Can you work these out from the model? Positions are in its coordinate system, mm. Coordinates: 2 decimals unless noted, no trailing zeros. Write each loop counter-clockwise with the first axis right and the second up, starting at its lowest first coordinate (ties: lowest second). Pieces come first, ordered by that corner, then holes. Notation, with made-up numbers: (83, 49.25) - (105, 49.25) arc R24 cw to (105, 70.25) - close; hole circle Ø5 at (31, 73). An arc over 180 degrees is marked (long way). Use one line per item in the form item = value. Start each with the question number.
(1) If we section it at C-C on y = -127.5: Please give me the cut outline in (x, z), then the cut area to 3 significant figures.
(2) If we section it at B-B on z = 0: Please give me the cut outline in (x, y), then the cut area to 3 significant figures.
(3) If we section it at A-A on x = 0: Please give me the cut outline in (y, z), then the cut area to 3 significant figures.
(4) If I drill on probe 1 along Z at (x, y) = (15, -39.45); probe 2 along Y at (x, z) = (-16.5, 14.5); probe 3 along Z at (x, y) = (-1.5, -140), over which ranges is the centre line in solid material (lowest first)? Write a range as from..to.
(5) For pin 1 Ø4 at (x, y) = (4, -64) entering from -Z; pin 2 Ø5 at (x, z) = (-16, -15) entering from +Y; pin 3 Ø2.5 at (x, z) = (-16, -15.5) entering from -Y; pin 4 Ø0.9 at (x, z) = (15.5, -15) entering from -Y, each with a flat end and sliding along its axis, tell me the tip position at first contact or that it passes through.
```python
from build123d import *

# Parameters (mm, degrees)
F0_W     = 42
F0_H     = 42
F1_DEPTH = 40
F2_R     = 4
F3_DEPTH = 325
F4_R     = 1.5
F5_DEPTH = 2


with BuildPart() as f1:
    # F0 (on Front) → F1 (new body)
    with BuildSketch(Plane.XZ):
        Rectangle(F0_W, F0_H)
    extrude(amount=F1_DEPTH)

    # F2 (on face) → F3 (join)
    with BuildSketch(Plane.XZ.offset(40)):
        Circle(F2_R)
    extrude(amount=F3_DEPTH)

    # F4 (on face) → F5 (cut)
    with BuildSketch(Plane.XZ.offset(40)):
        with Locations((-16, -15)):
            Circle(F4_R)
        with BuildLine():
            ThreePointArc((-17.5, 16), (-16, 14.5), (-14.5, 16))
            ThreePointArc((-14.5, 16), (-16, 17.5), (-17.5, 16))
        make_face()
        with Locations((15, -15)):
            Circle(F4_R)
        with Locations((15, 16)):
            Circle(F4_R)
    extrude(amount=-F5_DEPTH, mode=Mode.SUBTRACT)


solid = f1.part
```
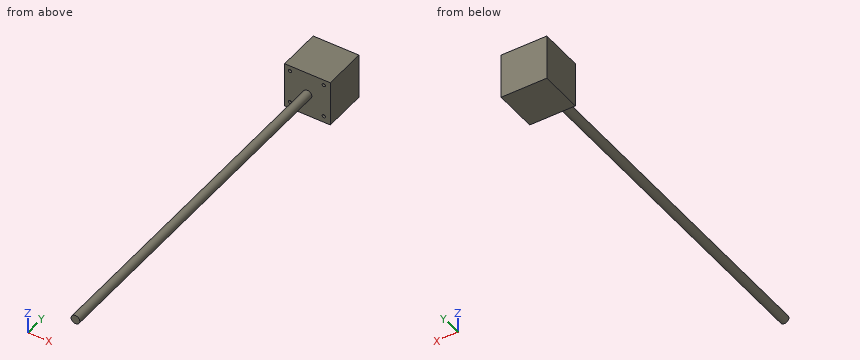
Reported:
q1.outline = circle Ø8 at (0, 0)
q1.area = 50.3 mm2
q2.outline = (-21, -40) - (-4, -40) - (-4, -365) - (4, -365) - (4, -40) - (21, -40) - (21, 0) - (-21, 0) - close
q2.area = 4,280 mm2
q3.outline = (-365, -4) - (-40, -4) - (-40, -21) - (0, -21) - (0, 21) - (-40, 21) - (-40, 4) - (-365, 4) - close
q3.area = 4,280 mm2
q4.probe_1 = -21..-16.5, -13.5..14.5, 17.5..21
q4.probe_2 = -40..0
q4.probe_3 = -3.71..3.71
q5.pin_1 = -3.46
q5.pin_2 = 0
q5.pin_3 = -40
q5.pin_4 = -38
